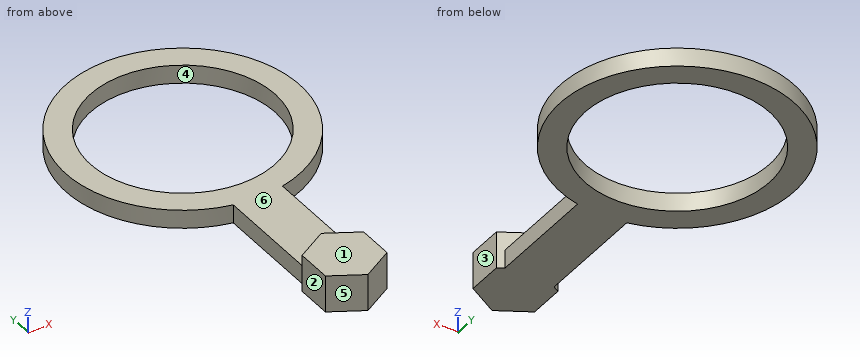
```python
from build123d import *

# Parameters (mm, degrees)
SKETCH1_R           = 19
SKETCH1_R_2         = 15
BOSS_EXTRUDE1_DEPTH = 3
BOSS_EXTRUDE2_DEPTH = 3


with BuildPart() as part:
    # Sketch1 → Boss-Extrude1 (new body)
    with BuildSketch(Plane.XY):
        Polygon((5, -2.886751346), (5, 2.886751346), (0, 5.773502692), (-5, 2.886751346), (-5, -2.886751346), (0, -5.773502692), align=None)
        with BuildLine():
            Line((-4, 3.464101615), (0, 5.773502692))
            Line((0, 5.773502692), (4, 3.464101615))
            Line((4, 3.464101615), (4, 21.425824379))
            ThreePointArc((4, 21.425824379), (0, 21), (-4, 21.425824379))
            Line((-4, 21.425824379), (-4, 3.464101615))
        make_face()
        with Locations((0, 40)):
            Circle(SKETCH1_R)
        with Locations((0, 40)):
            Circle(SKETCH1_R_2, mode=Mode.SUBTRACT)
    extrude(amount=BOSS_EXTRUDE1_DEPTH)

    # Sketch2 → Boss-Extrude2 (add)
    with BuildSketch(Plane.XY.offset(3)):
        Polygon((0, -5.773502692), (5, -2.886751346), (5, 2.886751346), (0, 5.773502692), (-5, 2.886751346), (-5, -2.886751346), align=None)
    extrude(amount=BOSS_EXTRUDE2_DEPTH)


solid = part.part
```
Part model, mm, in its own coordinate system. Face numbers are marked on the shaded views. A direction names the side the tool comes from. Give positions to 0.01 mm unless a question says otherwise; leave off trailing zeros. Loops run counter-clockwise (first coordinate to the right, second up) from the corner with the lowest first, then second, coordinate; pieces in that order, holes last. Notation, with made-up numbers: M 61,78.25 L 97,78.25 A24 cw 97,110.25 Z; hole C -32.5,55.25 d10. An arc over 180 degrees is marked long. Return JSON: item names as keys, results as strings.
1) Saw through at A-A, the plane y = 40. List the corners of the cut face in (x, z).
Calculated:
{"outline": "M -19,0 L -15,0 L -15,3 L -19,3 Z; M 15,0 L 19,0 L 19,3 L 15,3 Z"}
2) Saw through at B-B, the plane z = 1.95. List the corners of the cut face in (x, y).
Calculated:
{"outline": "M -5,-2.89 L 0,-5.77 L 5,-2.89 L 5,2.89 L 4,3.46 L 4,21.43 A19 ccw long -4,21.43 L -4,3.46 L -5,2.89 Z; hole C 0,40 d30"}
3) Saw through at D-D, the plane x = 14. List the corners of the cut face in (y, z).
Calculated:
{"outline": "M 27.15,0 L 34.61,0 L 34.61,3 L 27.15,3 Z; M 45.39,0 L 52.85,0 L 52.85,3 L 45.39,3 Z"}
4) Saw through at C-C, the plane x = -1. List the corners of the cut face in (y, z).
Calculated:
{"outline": "M -5.2,0 L 25.03,0 L 25.03,3 L 5.2,3 L 5.2,6 L -5.2,6 Z; M 54.97,0 L 58.97,0 L 58.97,3 L 54.97,3 Z"}
5) 3-axis set-ups, long thin cutter, end or side, ignore diameter. For the marked faces 1, 2 and 3: which of +Z, -Z, +X, -X, +Y, -Y reach the whole face in a straight line?
Calculated:
{"face 1": "+Z, +X, -X, +Y, -Y", "face 2": "+Z, -Z, -X, -Y", "face 3": "+Z, -Z, +X, -Y"}
6) Pull direction Y, two halves, no side cores. Call the marked faces 4, 5 and 6: released by +Y, released by -Y, zero draft, split by the parting line, or undercut.
Calculated:
{"face 4": "undercut", "face 5": "released by -Y", "face 6": "zero draft"}
7) Flat gauge pins, fed straight in: pin 1 Ø19 at (x, y) = (9.5, 33) entering from +Z; pin 2 Ø1 at (x, z) = (14.5, 1) entering from +Y; pin 3 Ø0.9 at (y, z) = (9.5, 1) entering from +X. Where does each tip first touch, or does it go through?
Calculated:
{"pin 1": "stops at z = 3", "pin 2": "stops at y = 52.85", "pin 3": "stops at x = 4"}
8) Drill centre lines: line 1 (X direction, y = -2, z = 2.9); line 2 (X direction, y = 41, z = 2.1); line 3 (X direction, y = 38, z = 0.45). Where is each one in solid material? Low to high.
Calculated:
{"line 1": "x = -5 to 5", "line 2": "x = -18.97 to -14.97, 14.97 to 18.97", "line 3": "x = -18.89 to -14.87, 14.87 to 18.89"}
